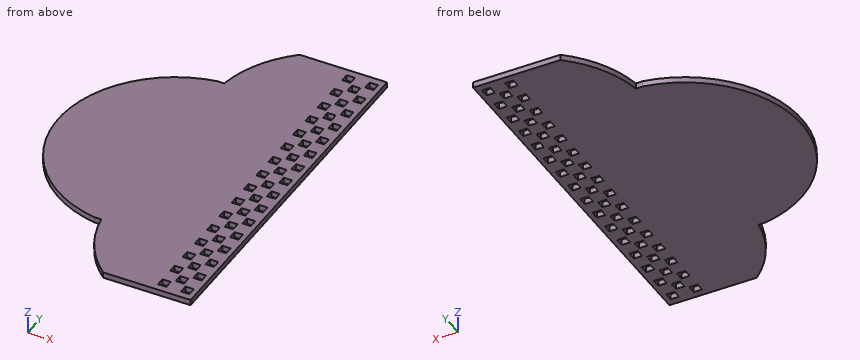
```python
from build123d import *

# Parameters (mm, degrees)
F0_W      = 24.13
F0_H      = 203.2
F0_W_2    = 4.6228
F0_H_2    = 4.6228
F1_DEPTH  = 3.175
F3_W      = 3.81
F3_H      = 127
F4_DEPTH  = 3.175
F5_W      = 24.13
F5_H      = 203.2
F6_DEPTH  = 3.175
F1_FACE_W = 203.2
F1_FACE_H = 3.175
F9_DEPTH  = 0.0254


with BuildPart() as f1:
    # F0 (on Top) → F1 (new body)
    with BuildSketch(Plane.XY):
        with Locations((0.48795, 36.187809)):
            Rectangle(F0_W, F0_H)
        with Locations((-5.27785, -59.112991)):
            Rectangle(F0_W_2, F0_H_2, mode=Mode.SUBTRACT)
        with Locations((-5.27785, -46.412991)):
            Rectangle(F0_W_2, F0_H_2, mode=Mode.SUBTRACT)
        with Locations((-5.27785, -33.712991)):
            Rectangle(F0_W_2, F0_H_2, mode=Mode.SUBTRACT)
        with Locations((-5.27785, -21.012991)):
            Rectangle(F0_W_2, F0_H_2, mode=Mode.SUBTRACT)
        with Locations((-5.27785, -8.312991)):
            Rectangle(F0_W_2, F0_H_2, mode=Mode.SUBTRACT)
        with Locations((-5.27785, 4.387009)):
            Rectangle(F0_W_2, F0_H_2, mode=Mode.SUBTRACT)
        with Locations((-5.27785, 17.087009)):
            Rectangle(F0_W_2, F0_H_2, mode=Mode.SUBTRACT)
        with Locations((-5.27785, 29.787009)):
            Rectangle(F0_W_2, F0_H_2, mode=Mode.SUBTRACT)
        with Locations((1.07215, -52.762991)):
            Rectangle(F0_W_2, F0_H_2, mode=Mode.SUBTRACT)
        with Locations((1.07215, -40.062991)):
            Rectangle(F0_W_2, F0_H_2, mode=Mode.SUBTRACT)
        with Locations((1.07215, -27.362991)):
            Rectangle(F0_W_2, F0_H_2, mode=Mode.SUBTRACT)
        with Locations((1.07215, -14.662991)):
            Rectangle(F0_W_2, F0_H_2, mode=Mode.SUBTRACT)
        with Locations((7.42215, -59.112991)):
            Rectangle(F0_W_2, F0_H_2, mode=Mode.SUBTRACT)
        with Locations((7.42215, -46.412991)):
            Rectangle(F0_W_2, F0_H_2, mode=Mode.SUBTRACT)
        with Locations((7.42215, -33.712991)):
            Rectangle(F0_W_2, F0_H_2, mode=Mode.SUBTRACT)
        with Locations((7.42215, -21.012991)):
            Rectangle(F0_W_2, F0_H_2, mode=Mode.SUBTRACT)
        with Locations((1.07215, -1.962991)):
            Rectangle(F0_W_2, F0_H_2, mode=Mode.SUBTRACT)
        with Locations((1.07215, 10.737009)):
            Rectangle(F0_W_2, F0_H_2, mode=Mode.SUBTRACT)
        with Locations((1.07215, 23.437009)):
            Rectangle(F0_W_2, F0_H_2, mode=Mode.SUBTRACT)
        with Locations((1.07215, 36.137009)):
            Rectangle(F0_W_2, F0_H_2, mode=Mode.SUBTRACT)
        with Locations((7.42215, -8.312991)):
            Rectangle(F0_W_2, F0_H_2, mode=Mode.SUBTRACT)
        with Locations((7.42215, 4.387009)):
            Rectangle(F0_W_2, F0_H_2, mode=Mode.SUBTRACT)
        with Locations((7.42215, 17.087009)):
            Rectangle(F0_W_2, F0_H_2, mode=Mode.SUBTRACT)
        with Locations((7.42215, 29.787009)):
            Rectangle(F0_W_2, F0_H_2, mode=Mode.SUBTRACT)
        with Locations((-5.27785, 42.487009)):
            Rectangle(F0_W_2, F0_H_2, mode=Mode.SUBTRACT)
        with Locations((-5.27785, 55.187009)):
            Rectangle(F0_W_2, F0_H_2, mode=Mode.SUBTRACT)
        with Locations((-5.27785, 67.887009)):
            Rectangle(F0_W_2, F0_H_2, mode=Mode.SUBTRACT)
        with Locations((-5.27785, 80.587009)):
            Rectangle(F0_W_2, F0_H_2, mode=Mode.SUBTRACT)
        with Locations((-5.27785, 93.287009)):
            Rectangle(F0_W_2, F0_H_2, mode=Mode.SUBTRACT)
        with Locations((-5.27785, 105.987009)):
            Rectangle(F0_W_2, F0_H_2, mode=Mode.SUBTRACT)
        with Locations((-5.27785, 118.687009)):
            Rectangle(F0_W_2, F0_H_2, mode=Mode.SUBTRACT)
        with Locations((-5.27785, 131.387009)):
            Rectangle(F0_W_2, F0_H_2, mode=Mode.SUBTRACT)
        with Locations((1.07215, 48.837009)):
            Rectangle(F0_W_2, F0_H_2, mode=Mode.SUBTRACT)
        with Locations((1.07215, 61.537009)):
            Rectangle(F0_W_2, F0_H_2, mode=Mode.SUBTRACT)
        with Locations((1.07215, 74.237009)):
            Rectangle(F0_W_2, F0_H_2, mode=Mode.SUBTRACT)
        with Locations((1.07215, 86.937009)):
            Rectangle(F0_W_2, F0_H_2, mode=Mode.SUBTRACT)
        with Locations((7.42215, 42.487009)):
            Rectangle(F0_W_2, F0_H_2, mode=Mode.SUBTRACT)
        with Locations((7.42215, 55.187009)):
            Rectangle(F0_W_2, F0_H_2, mode=Mode.SUBTRACT)
        with Locations((7.42215, 67.887009)):
            Rectangle(F0_W_2, F0_H_2, mode=Mode.SUBTRACT)
        with Locations((7.42215, 80.587009)):
            Rectangle(F0_W_2, F0_H_2, mode=Mode.SUBTRACT)
        with Locations((1.07215, 99.637009)):
            Rectangle(F0_W_2, F0_H_2, mode=Mode.SUBTRACT)
        with Locations((1.07215, 112.337009)):
            Rectangle(F0_W_2, F0_H_2, mode=Mode.SUBTRACT)
        with Locations((1.07215, 125.037009)):
            Rectangle(F0_W_2, F0_H_2, mode=Mode.SUBTRACT)
        with Locations((7.42215, 93.287009)):
            Rectangle(F0_W_2, F0_H_2, mode=Mode.SUBTRACT)
        with Locations((7.42215, 105.987009)):
            Rectangle(F0_W_2, F0_H_2, mode=Mode.SUBTRACT)
        with Locations((7.42215, 118.687009)):
            Rectangle(F0_W_2, F0_H_2, mode=Mode.SUBTRACT)
        with Locations((7.42215, 131.387009)):
            Rectangle(F0_W_2, F0_H_2, mode=Mode.SUBTRACT)
    extrude(amount=F1_DEPTH)

    # F2: F1 across face


with BuildPart() as f1_1:
    add(f1.part)
    add(f1.part.mirror(Plane(origin=(-11.57705, 36.187809, 1.5875), x_dir=(0, -1, 0), z_dir=(-1, 0, 0))))

    # F3 (on face) → F4 (join)
    with BuildSketch(Plane(origin=(0, 0, 0), x_dir=(1, 0, 0), z_dir=(0, 0, -1))):
        with BuildLine():
            Line((-35.70705, -137.787809), (-35.70705, 65.412191))
            ThreePointArc((-35.70705, 65.412191), (-49.82872, 48.296246), (-57.04305, 27.312191))
            Line((-57.04305, 27.312191), (-57.04305, -99.687809))
            ThreePointArc((-57.04305, -99.687809), (-49.82872, -120.671864), (-35.70705, -137.787809))
        make_face()
        with Locations((-58.94805, -36.187809)):
            Rectangle(F3_W, F3_H)
        with BuildLine():
            Line((-60.85305, -99.687809), (-60.85305, 27.312191))
            ThreePointArc((-60.85305, 27.312191), (-114.585848, -36.187809), (-60.85305, -99.687809))
        make_face()
    extrude(amount=-F4_DEPTH)

    # F5 (on face) → F6 (join)
    with BuildSketch(Plane.XY.offset(3.175)):
        with Locations((-23.64205, 36.187809)):
            Rectangle(F5_W, F5_H)
    extrude(amount=-F6_DEPTH)

    # F1_face (on face) → F9 (cut)
    with BuildSketch(Plane(origin=(12.55295, 36.187809, 1.5875), x_dir=(0, 1, 0), z_dir=(1, 0, 0))):
        Rectangle(F1_FACE_W, F1_FACE_H)
    extrude(amount=-F9_DEPTH, mode=Mode.SUBTRACT)


solid = f1_1.part
```
CAD build for the part. Positions are in the model's coordinates, mm. Round coordinates to 2 decimals unless told otherwise and drop trailing zeros. Order: outer loops, then holes, each group sorted by start corner. A loop starts at its lowest first (then second) coordinate and runs counter-clockwise, first axis right, second up. Notation, with made-up numbers: (12.25, 37) - (33.25, 37) arc R25 cw to (33.25, 65) - close; hole circle Ø11 at (-25, -36.5). An arc over 180 degrees is marked (long way). Use CSV: the item, a comma, the result in double quotes. Start each with the question number.
1) Wall check: L1, parallel to X at y = 19, z = 1.8; L2, parallel to X at y = -48.5, z = 0.9; L3, parallel to X at y = -14.5, z = 2.9. Give the ranges that are in metal, low to high. Write a range as [from, to].
2) Saw through at B-B (z = 2.05). Count the separate pieces of the cut face and the enclosed holes in it, and give its area (3 significant figures).
3) Saw through at D-D (x = -49). List the corners of the cut face in (y, z) (3 decimals).
4) Saw through at C-C (x = -64). List the corners of the cut face in (y, z) (3 decimals).
5) Saw through at A-A (y = 30). List the corners of the cut face in (x, z) (3 decimals), and give its area (3 significant figures).
Values follow:
1,L1,"x = [-112.25, -7.59], [-2.97, 5.11], [9.73, 12.53]"
1,L2,"x = [-49.71, -7.59], [-2.97, 5.11], [9.73, 12.53]"
1,L3,"x = [-89.9, -1.24], [3.38, 12.53]"
2,separate pieces,"1"
2,enclosed holes,"47"
2,area,"18,200 mm2"
3,outline,"(-49.731, 0) - (122.107, 0) - (122.107, 3.175) - (-49.731, 3.175) - close"
4,outline,"(-26.703, 0) - (99.079, 0) - (99.079, 3.175) - (-26.703, 3.175) - close"
5,outline,"(-114.288, 0) - (-7.589, 0) - (-7.589, 3.175) - (-114.288, 3.175) - close; (-2.966, 0) - (5.111, 0) - (5.111, 3.175) - (-2.966, 3.175) - close; (9.734, 0) - (12.528, 0) - (12.528, 3.175) - (9.734, 3.175) - close"
5,area,"373 mm2"
